from build123d import *

# Parameters (mm, degrees)
SKETCH2_W           = 29
SKETCH2_H           = 29
BOSS_EXTRUDE3_DEPTH = 23
SHELL3_T            = -4.5
SKETCH7_R           = 4.25
CUT_EXTRUDE9_DEPTH  = 3
SKETCH10_R          = 4.25
CUT_EXTRUDE10_DEPTH = 3
CUT_EXTRUDE11_START = -3
SKETCH9_R           = 4.25
CUT_EXTRUDE11_DEPTH = 3
CUT_EXTRUDE12_START = -3
SKETCH8_R           = 4.25
CUT_EXTRUDE12_DEPTH = 3
SKETCH12_R          = 2.5
CUT_EXTRUDE13_DEPTH = 39.813018756
SKETCH13_R          = 2.5
CUT_EXTRUDE14_DEPTH = 11.5
CUT_EXTRUDE15_START = -11.5
SKETCH14_R          = 2.5
CUT_EXTRUDE15_DEPTH = 11.5


with BuildPart() as part:
    # Sketch2 → Boss-Extrude3 (new body)
    with BuildSketch(Plane.XY):
        with Locations((2.862327752, -2.483638693)):
            Rectangle(SKETCH2_W, SKETCH2_H)
    extrude(amount=BOSS_EXTRUDE3_DEPTH)

    # Shell3
    shell3_openings = [part.faces().sort_by_distance(p)[0] for p in [
        (2.862327752, -2.483638693, 23),
    ]]
    offset(amount=SHELL3_T, openings=shell3_openings, kind=Kind.INTERSECTION)

    # Sketch7 → Cut-Extrude9 (cut)
    with BuildSketch(Plane(origin=(0, -16.983638693, 0), x_dir=(-1, 0, 0), z_dir=(0, -1, 0))):
        with Locations(Location((-2.862327752, -11.5, 0), (0, 0, 90))):
            Circle(SKETCH7_R)
    extrude(amount=-CUT_EXTRUDE9_DEPTH, mode=Mode.SUBTRACT)

    # Sketch10 → Cut-Extrude10 (cut)
    with BuildSketch(Plane(origin=(17.362327752, 0, 0), x_dir=(0, 0, -1), z_dir=(1, 0, 0))):
        with Locations(Location((-11.5, -2.483638693, 0), (0, 0, 90))):
            Circle(SKETCH10_R)
    extrude(amount=-CUT_EXTRUDE10_DEPTH, mode=Mode.SUBTRACT)

    # Sketch9 → Cut-Extrude11 (cut)
    with BuildSketch(Plane(origin=(0, 12.016361307, 0), x_dir=(1, 0, 0), z_dir=(0, 1, 0)).offset(CUT_EXTRUDE11_START)):
        with Locations(Location((2.862327752, -11.5, 0), (0, 0, 90))):
            Circle(SKETCH9_R)
    extrude(amount=CUT_EXTRUDE11_DEPTH, mode=Mode.SUBTRACT)

    # Sketch8 → Cut-Extrude12 (cut)
    with BuildSketch(Plane.ZY.offset(11.637672248).offset(CUT_EXTRUDE12_START)):
        with Locations(Location((11.5, -2.483638693, 0), (0, 0, 90))):
            Circle(SKETCH8_R)
    extrude(amount=CUT_EXTRUDE12_DEPTH, mode=Mode.SUBTRACT)

    # Sketch12 → Cut-Extrude13 (cut, through all)
    with BuildSketch(Plane(origin=(0, 9.016361307, 0), x_dir=(1, 0, 0), z_dir=(0, 1, 0))):
        with Locations(Location((2.862327752, -11.5, 0), (0, 0, 270))):
            Circle(SKETCH12_R)
    extrude(amount=-CUT_EXTRUDE13_DEPTH, mode=Mode.SUBTRACT)

    # Sketch13 → Cut-Extrude14 (cut)
    with BuildSketch(Plane(origin=(14.362327752, 0, 0), x_dir=(0, 0, -1), z_dir=(1, 0, 0))):
        with Locations(Location((-11.5, -2.483638693, 0), (0, 0, 90))):
            Circle(SKETCH13_R)
    extrude(amount=-CUT_EXTRUDE14_DEPTH, mode=Mode.SUBTRACT)

    # Sketch14 → Cut-Extrude15 (cut)
    with BuildSketch(Plane.ZY.offset(8.637672248).offset(CUT_EXTRUDE15_START)):
        with Locations(Location((11.5, -2.483638693, 0), (0, 0, 90))):
            Circle(SKETCH14_R)
    extrude(amount=CUT_EXTRUDE15_DEPTH, mode=Mode.SUBTRACT)


solid = part.part
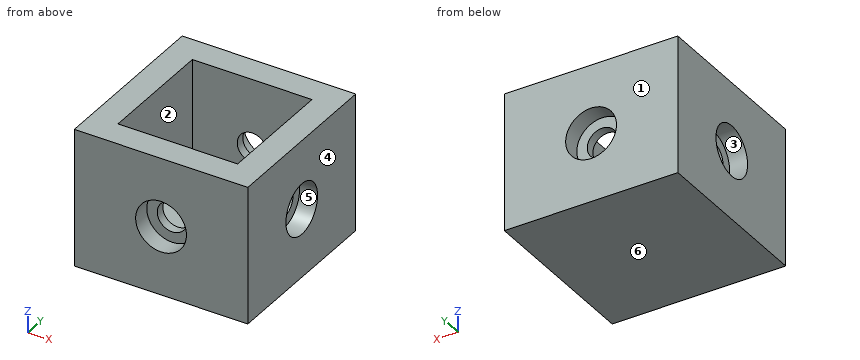
Design review of the part built by this model. Coordinates are the model's own, in mm. Face numbers are marked on the shaded views. A direction names the side the tool comes from. Coordinates: 2 decimals unless noted, no trailing zeros. Loops run counter-clockwise (first coordinate to the right, second up) from the corner with the lowest first, then second, coordinate; pieces in that order, holes last. Notation, with made-up numbers: M -24.5,5 L 22.5,5 A31 ccw 22.5,37 Z; hole C 40.25,-20.5 d2. An arc over 180 degrees is marked long. Use one line per item in the form item = value.
(1) For the marked faces 1 and 2, list the 3-axis set-ups (+Z, -Z, +X, -X, +Y, -Y) from which the entire face can be reached by the end or side of a thin tool; tool diameter is ignored.
Return value:
face_1 = +Z, -Z, +X, -X, +Y
face_2 = +Z
(2) Consider section B-B (z = 16.75). Write out the cut boundary in (x, y).
Return value:
outline = M -11.64,-16.98 L 17.36,-16.98 L 17.36,12.02 L -11.64,12.02 Z; hole M -7.14,-12.48 L 12.86,-12.48 L 12.86,7.52 L -7.14,7.52 Z
(3) Clearance check with flat-ended pins moving along their axes: P1, Ø9.5, axis at y = -4, z = 11.5, coming from the -X side; P2, Ø6.5, axis at y = -2.48, z = 11.5, coming from the -X side; P3, Ø1.5, axis at x = -4, y = -7, coming from the +Z side; P4, Ø6, axis at y = -2.48, z = 11.5, coming from the +X side. State where each tip first meets the part, or that it passes through.
Return value:
P1 = -11.64
P2 = -8.64
P3 = 4.5
P4 = 14.36
(4) For line 1 along X through (y, z) = (7.25, 22); line 2 along Y through (x, z) = (-8.25, 11.5); line 3 along X through (y, z) = (10.5, 11.5), list the stretches that pass through material, from the lowest coordinate up. Write a range as from..to.
Return value:
line_1 = -11.64..-7.14, 12.86..17.36
line_2 = -16.98..-4.98, 0.02..12.02
line_3 = -11.64..-1.39, 7.11..17.36
(5) Consider section C-C (y = 2.75). Write out the cut boundary in (x, z).
Return value:
outline = M -11.64,0 L 17.36,0 L 17.36,23 L 12.86,23 L 12.86,4.5 L -7.14,4.5 L -7.14,23 L -11.64,23 Z
(6) Consider section D-D (x = -6.5). Write out the cut boundary in (y, z).
Return value:
outline = M -16.98,0 L 12.02,0 L 12.02,23 L 7.52,23 L 7.52,4.5 L -12.48,4.5 L -12.48,23 L -16.98,23 Z
(7) Draft analysis for pull direction Z (two halves, no side actions). For the marked faces 3, 4, 5 and 6, state which applies: pulls with the +Z half, pulls with the -Z half, needs draft (parallel to the pull), parting line crosses it, or undercut.
Return value:
face_3 = undercut
face_4 = needs draft
face_5 = undercut
face_6 = pulls with the -Z half
(8) Consider section A-A (x = 3.75). Write out the cut boundary in (y, z).
Return value:
outline = M -16.98,0 L 12.02,0 L 12.02,7.34 L 9.02,7.34 L 9.02,9.16 L 7.52,9.16 L 7.52,4.5 L -12.48,4.5 L -12.48,9.16 L -13.98,9.16 L -13.98,7.34 L -16.98,7.34 Z; M -16.98,15.66 L -13.98,15.66 L -13.98,13.84 L -12.48,13.84 L -12.48,23 L -16.98,23 Z; M 7.52,13.84 L 9.02,13.84 L 9.02,15.66 L 12.02,15.66 L 12.02,23 L 7.52,23 Z
